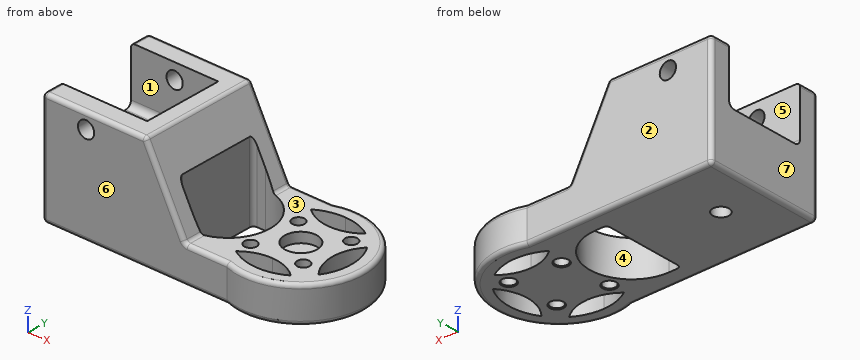
from build123d import *

# Parameters (mm, degrees)
ESQUISSE4_R                   = 13.9
ESQUISSE4_R_2                 = 1.55
BOSS_EXTRU_3_DEPTH            = 4.5
ESQUISSE7_R                   = 15.9
ESQUISSE7_R_2                 = 13.9
BOSS_EXTRU_7_DEPTH            = 9
BOSS_EXTRU_8_DEPTH            = 30
ENL_V_START                   = -4.5
ENL_V_MAT_EXTRU_12_OUTLINE_R  = 1.55
ENL_V_MAT_EXTRU_12_DEPTH      = 9
TROU_TARAUD_M32_D             = 2.5
TROU_TARAUD_M32_DEPTH         = 36
TROU_TARAUD_M32_CSINK_D       = 3.5
TROU_TARAUD_M32_CSINK_ANGLE   = 90
ENL_V_MAT_EXTRU_1_DEPTH       = 22
ESQUISSE13_R                  = 2.05
ENL_V_MAT_EXTRU_4_DEPTH       = 69.045108798
ESQUISSE15_R                  = 2.05
ENL_V_MAT_EXTRU_5_DEPTH       = 66.052954056
ENL_V_MAT_EXTRU_6_DEPTH       = 77.342234353
ESQUISSE24_R                  = 4.05
ENL_V_MAT_EXTRU_9_DEPTH       = 2.5
TROU_TARAUD_M33_D             = 2.5
TROU_TARAUD_M33_DEPTH         = 28.24245014
TROU_TARAUD_M33_CSINK_D       = 3.5
TROU_TARAUD_M33_CSINK_ANGLE   = 90
CONG_2_R                      = 1
ENL_V_MAT_EXTRU_13_DEPTH      = 58.499206362
ENL_V_MAT_EXTRU_13_DEPTH_BACK = 58.499206362
CONG_3_R                      = 1
CONG_4_R                      = 1


# Read off the part's stored shape, not the designer's step: Enlèv. mat.-Extru.12
with BuildPart() as part:
    # Esquisse4 → Boss.-Extru.3 (new, symmetric)
    with BuildSketch(Plane.XY):
        Circle(ESQUISSE4_R)
        with Locations((-6.717514421, -6.717514421)):
            Circle(ESQUISSE4_R_2, mode=Mode.SUBTRACT)
        with Locations((6.717514421, 6.717514421)):
            Circle(ESQUISSE4_R_2, mode=Mode.SUBTRACT)
        with Locations((-5.656854249, 5.656854249)):
            Circle(ESQUISSE4_R_2, mode=Mode.SUBTRACT)
        with Locations((5.656854249, -5.656854249)):
            Circle(ESQUISSE4_R_2, mode=Mode.SUBTRACT)
        with BuildLine():
            ThreePointArc((-10.594734512, 6.911881121), (-12.65, 0), (-10.594734512, -6.911881121))
            ThreePointArc((-10.594734512, -6.911881121), (-7.999175124, 0), (-10.594734512, 6.911881121))
        make_face(mode=Mode.SUBTRACT)
        with BuildLine():
            ThreePointArc((6.911881121, -10.594734512), (0, -7.999175124), (-6.911881121, -10.594734512))
            ThreePointArc((-6.911881121, -10.594734512), (0, -12.65), (6.911881121, -10.594734512))
        make_face(mode=Mode.SUBTRACT)
        with BuildLine():
            ThreePointArc((-6.911881121, 10.594734512), (0, 7.999175124), (6.911881121, 10.594734512))
            ThreePointArc((6.911881121, 10.594734512), (0, 12.65), (-6.911881121, 10.594734512))
        make_face(mode=Mode.SUBTRACT)
        with BuildLine():
            ThreePointArc((10.594734512, 6.911881121), (7.999175124, 0), (10.594734512, -6.911881121))
            ThreePointArc((10.594734512, -6.911881121), (12.65, 0), (10.594734512, 6.911881121))
        make_face(mode=Mode.SUBTRACT)
    extrude(amount=BOSS_EXTRU_3_DEPTH, both=True)

    # Esquisse7 → Boss.-Extru.7 (add)
    with BuildSketch(Plane.XY.offset(4.5)):
        Circle(ESQUISSE7_R)
        Circle(ESQUISSE7_R_2, mode=Mode.SUBTRACT)
    extrude(amount=-BOSS_EXTRU_7_DEPTH)

    # Esquisse6 → Boss.-Extru.8 (add)
    with BuildSketch(Plane(origin=(0, -15, 0), x_dir=(1, 0, 0), z_dir=(0, 1, 0))):
        Polygon((-51.798424989, -31.5), (-29.798424989, -31.5), (-15.9, -4.5), (0, -4.5), (0, 4.5), (-15.9, 4.5), (-51.798424989, 4.5), align=None)
    extrude(amount=BOSS_EXTRU_8_DEPTH)

    # Enlèv. mat.-Extru.12 outline → Enlèv. mat.-Extru.12 (cut)
    with BuildSketch(Plane.XY.offset(ENL_V_START)):
        with BuildLine():
            ThreePointArc((0, 12.65), (-3.605489456, 12.125301884), (-6.911881121, 10.594734512))
            ThreePointArc((-6.911881121, 10.594734512), (-6.773099648, 10.475509721), (-6.632262004, 10.358720998))
            ThreePointArc((-6.632262004, 10.358720998), (-6.631896353, 10.3589551), (-6.631530694, 10.359189189))
            ThreePointArc((-6.631530694, 10.359189189), (-3.519338467, 8.607363508), (0, 8))
            Line((0, 8), (0, 12.65))
        make_face()
        with BuildLine():
            ThreePointArc((-6.911881121, -10.594734512), (-3.605489456, -12.125301884), (0, -12.65))
            Line((0, -12.65), (0, -8))
            ThreePointArc((0, -8), (-3.519338467, -8.607363508), (-6.631530694, -10.359189189))
            ThreePointArc((-6.631530694, -10.359189189), (-6.631896353, -10.3589551), (-6.632262004, -10.358720998))
            ThreePointArc((-6.632262004, -10.358720998), (-6.773099648, -10.475509721), (-6.911881121, -10.594734512))
        make_face()
        with BuildLine():
            ThreePointArc((-10.358720998, 6.632262004), (-10.475509721, 6.773099648), (-10.594734512, 6.911881121))
            ThreePointArc((-10.594734512, 6.911881121), (-12.65, 0), (-10.594734512, -6.911881121))
            ThreePointArc((-10.594734512, -6.911881121), (-10.475509721, -6.773099648), (-10.358720998, -6.632262004))
            ThreePointArc((-10.358720998, -6.632262004), (-10.3589551, -6.631896353), (-10.359189189, -6.631530694))
            ThreePointArc((-10.359189189, -6.631530694), (-8, 0), (-10.359189189, 6.631530694))
            ThreePointArc((-10.359189189, 6.631530694), (-10.3589551, 6.631896353), (-10.358720998, 6.632262004))
        make_face()
        with Locations((-6.717514421, -6.717514421)):
            Circle(ENL_V_MAT_EXTRU_12_OUTLINE_R)
        with Locations((-5.656854249, 5.656854249)):
            Circle(ENL_V_MAT_EXTRU_12_OUTLINE_R)
    extrude(amount=ENL_V_MAT_EXTRU_12_DEPTH, mode=Mode.SUBTRACT)

    # Trou taraudé M32
    with Locations(Plane(origin=(5.656854249, -5.656854249, -4.5), x_dir=(-1, 0, 0), z_dir=(0, 0, -1))):
        with Locations((0, 0), (-1.060660172, 12.37436867)):
            CounterSinkHole(TROU_TARAUD_M32_D / 2, TROU_TARAUD_M32_CSINK_D / 2, depth=TROU_TARAUD_M32_DEPTH, counter_sink_angle=TROU_TARAUD_M32_CSINK_ANGLE)

    # Esquisse8 → Enlèv. mat.-Extru.1 (cut)
    with BuildSketch(Plane.ZY.offset(51.798424989)):
        with BuildLine():
            Line((28.34, 10.05), (11.34, 10.05))
            ThreePointArc((11.34, 10.05), (10.279339828, 9.610660172), (9.84, 8.55))
            Line((9.84, 8.55), (9.84, -8.55))
            ThreePointArc((9.84, -8.55), (10.279339828, -9.610660172), (11.34, -10.05))
            Line((11.34, -10.05), (28.34, -10.05))
            ThreePointArc((28.34, -10.05), (29.400660172, -9.610660172), (29.84, -8.55))
            Line((29.84, -8.55), (29.84, 8.55))
            ThreePointArc((29.84, 8.55), (29.400660172, 9.610660172), (28.34, 10.05))
        make_face()
    extrude(amount=-ENL_V_MAT_EXTRU_1_DEPTH, mode=Mode.SUBTRACT)

    # Esquisse13 → Enlèv. mat.-Extru.4 (cut, through all)
    with BuildSketch(Plane.XZ.offset(15)):
        with Locations(Location((-40.798424989, 19.84, 0), (0, 0, 270))):
            Circle(ESQUISSE13_R)
    extrude(amount=-ENL_V_MAT_EXTRU_4_DEPTH, mode=Mode.SUBTRACT)

    # Esquisse15 → Enlèv. mat.-Extru.5 (cut, through all)
    with BuildSketch(Plane(origin=(0, 0, -4.5), x_dir=(-1, 0, 0), z_dir=(0, 0, -1))):
        with Locations((40.798424989, 0)):
            Circle(ESQUISSE15_R)
    extrude(amount=-ENL_V_MAT_EXTRU_5_DEPTH, mode=Mode.SUBTRACT)

    # Esquisse16 → Enlèv. mat.-Extru.6 (cut, through all)
    with BuildSketch(Plane.ZY.offset(51.798424989)):
        Polygon((23.74245014, 10.05), (23.74245014, -10.05), (23.74245014, -15), (31.5, -15), (31.5, 15), (23.74245014, 15), align=None)
    extrude(amount=-ENL_V_MAT_EXTRU_6_DEPTH, mode=Mode.SUBTRACT)

    # Esquisse24 → Enlèv. mat.-Extru.9 (cut)
    with BuildSketch(Plane.XY.offset(4.5)):
        Circle(ESQUISSE24_R)
    extrude(amount=-ENL_V_MAT_EXTRU_9_DEPTH, mode=Mode.SUBTRACT)

    # Trou taraudé M33
    with Locations(Plane(origin=(0, 0, -4.5), x_dir=(-1, 0, 0), z_dir=(0, 0, -1))):
        with Locations((6.717514421, -6.717514421), (5.656854249, 5.656854249)):
            CounterSinkHole(TROU_TARAUD_M33_D / 2, TROU_TARAUD_M33_CSINK_D / 2, depth=TROU_TARAUD_M33_DEPTH, counter_sink_angle=TROU_TARAUD_M33_CSINK_ANGLE)

    # Congé2
    cong_2_edges = [part.edges().sort_by_distance(p)[0] for p in [
        (-20.852587961, -15, 14.12122507),
        (-20.852587961, 15, 14.12122507),
        (-38.801800455, 15, 23.74245014),
        (-25.805175921, 0, 23.74245014),
        (-38.801800455, -15, 23.74245014),
        (15.9, 0, -4.5),
        (15.9, 0, 4.5),
        (-15.9, 0, 4.5),
        (-10.586759375, -15, 4.5),
        (-28.535971869, -15, -4.5),
        (-51.798424989, 0, -4.5),
        (-28.535971869, 15, -4.5),
        (-10.586759375, 15, 4.5),
    ]]
    fillet(cong_2_edges, radius=CONG_2_R)

    # Esquisse27 → Enlèv. mat.-Extru.13 (cut, two sides: drawn at the far end of the back side and taken through both)
    with BuildSketch(Plane.XY.offset(4.5).offset(-ENL_V_MAT_EXTRU_13_DEPTH_BACK)):
        with BuildLine():
            Line((-18.31885198, -10.5), (-21.396528806, -10.5))
            Line((-21.396528806, -10.5), (-21.396528806, 10.5))
            Line((-21.396528806, 10.5), (-18.31885198, 10.5))
            ThreePointArc((-18.31885198, 10.5), (-7.81885198, 0), (-18.31885198, -10.5))
        make_face()
    extrude(amount=ENL_V_MAT_EXTRU_13_DEPTH + ENL_V_MAT_EXTRU_13_DEPTH_BACK, mode=Mode.SUBTRACT)

    # Congé3
    cong_3_edges = [part.edges().sort_by_distance(p)[0] for p in [
        (-21.396528806, 10.5, 5.338960274),
        (-21.396528806, -10.5, 5.338960274),
    ]]
    fillet(cong_3_edges, radius=CONG_3_R)

    # Congé4
    # the kernel refuses this fillet: 1 mm, written as the material it takes off along each edge
    with BuildSketch(Plane(origin=(-50.798424989, 14, -3.5), x_dir=(-1, 0, 0), z_dir=(0, 1, 0))) as cong_4_piece_1_section:
        Polygon((0, 0), (CONG_4_R, 0), (CONG_4_R, -CONG_4_R), (0, -CONG_4_R), align=None)
    cong_4_piece_1 = extrude(amount=CONG_4_R, mode=Mode.PRIVATE)
    cong_4_piece_1 = cong_4_piece_1 - Plane(origin=(-50.798424989, 14, -3.5), x_dir=(0.7071067811865477, 0, 0.7071067811865475), z_dir=(0, 1, 0)) * Sphere(CONG_4_R, mode=Mode.PRIVATE)
    add(cong_4_piece_1, mode=Mode.SUBTRACT)
    with BuildSketch(Plane(origin=(-50.798424989, -14, -3.5), x_dir=(-1, 0, 0), z_dir=(0, -1, 0))) as cong_4_piece_2_section:
        Polygon((0, 0), (CONG_4_R, 0), (CONG_4_R, CONG_4_R), (0, CONG_4_R), align=None)
    cong_4_piece_2 = extrude(amount=CONG_4_R, mode=Mode.PRIVATE)
    cong_4_piece_2 = cong_4_piece_2 - Plane(origin=(-50.798424989, -14, -3.5), x_dir=(0.7071067811865477, 0, 0.7071067811865475), z_dir=(0, -1, 0)) * Sphere(CONG_4_R, mode=Mode.PRIVATE)
    add(cong_4_piece_2, mode=Mode.SUBTRACT)
    with BuildSketch(Plane(origin=(-51.798424989, -14, 23.74245014), x_dir=(1, 0, 0), z_dir=(0, 1, 0)), Plane(origin=(-51.798424989, 7.55, 23.74245014), x_dir=(1, 0, 0), z_dir=(0, 1, 0))) as cong_4_piece_3:
        with BuildLine():
            CenterArc((CONG_4_R, CONG_4_R), CONG_4_R, 180, 90)
            Line((0, CONG_4_R), (0, 0))
            Line((0, 0), (CONG_4_R, 0))
        make_face()
    extrude(amount=6.45, mode=Mode.SUBTRACT)
    with BuildSketch(Plane(origin=(-51.798424989, -15, -3.5), x_dir=(1, 0, 0), z_dir=(0, 0, 1))) as cong_4_piece_4:
        with BuildLine():
            CenterArc((CONG_4_R, CONG_4_R), CONG_4_R, 180, 90)
            Line((0, CONG_4_R), (0, 0))
            Line((0, 0), (CONG_4_R, 0))
        make_face()
    extrude(amount=26.24245014, mode=Mode.SUBTRACT)
    with BuildSketch(Plane(origin=(-51.798424989, 15, -3.5), x_dir=(1, 0, 0), z_dir=(0, 0, 1))) as cong_4_piece_5:
        with BuildLine():
            CenterArc((CONG_4_R, -CONG_4_R), CONG_4_R, 90, 90)
            Line((0, -CONG_4_R), (0, 0))
            Line((0, 0), (CONG_4_R, 0))
        make_face()
    extrude(amount=26.24245014, mode=Mode.SUBTRACT)
    with BuildSketch(Plane(origin=(-51.798424989, 14, 22.74245014), x_dir=(0, 0, 1), z_dir=(0, -1, 0))) as cong_4_piece_6:
        with BuildLine():
            CenterArc((1 - CONG_4_R, -CONG_4_R), CONG_4_R, 0, 90)
            Line((1, -CONG_4_R), (1, 0))
            Line((1, 0), (1 - CONG_4_R, 0))
        make_face()
    revolve(axis=Axis((-51.798424989, 14, 22.74245014), (-1, 0, 0)), revolution_arc=90, mode=Mode.SUBTRACT)
    with BuildSketch(Plane(origin=(-51.798424989, -14, 22.74245014), x_dir=(0, 0, 1), z_dir=(0, 1, 0))) as cong_4_piece_7:
        with BuildLine():
            CenterArc((1 - CONG_4_R, CONG_4_R), CONG_4_R, 270, 90)
            Line((1 - CONG_4_R, 0), (1, 0))
            Line((1, 0), (1, CONG_4_R))
        make_face()
    revolve(axis=Axis((-51.798424989, -14, 22.74245014), (1, 0, 0)), revolution_arc=90, mode=Mode.SUBTRACT)


solid = part.part
Can you work these out from the model? Positions are in its coordinate system, mm. Face numbers are marked on the shaded views. A direction names the side the tool comes from. Give positions to 0.01 mm unless a question says otherwise; leave off trailing zeros. Loops run counter-clockwise (first coordinate to the right, second up) from the corner with the lowest first, then second, coordinate; pieces in that order, holes last. Notation, with made-up numbers: (22, -12.5) -> (45, -12.5) arc R25 cw to (45, 9.5) -> close; hole circle Ø1 at (-6.5, 10). An arc over 180 degrees is marked (long way). Write item = value, one per line.
1) I need wall thicknesses on L1, parallel to X at y = 4.5, z = -1.25; L2, parallel to Y at x = 6, z = 1.5; L3, parallel to Y at x = -39.5, z = 12. Which ranges of each line are inside material? Lowest first, please. Write a range as from..to.
Check result:
L1 = -51.8..-21.4, -8.83..-6.69, -4.63..9.01, 11.82..15.25
L2 = -14.72..-11.14, -9.88..-7.17, -4.15..5.34, 8.09..9.88, 11.14..14.72
L3 = -15..-10.05, 10.05..15
2) Suppose I cut it at B-B on x = -13. Write out the boundary of the cut face in (y, z).
Check result:
outline = (-15, -3.5) arc R1 ccw to (-14, -4.5) -> (-9.05, -4.5) -> (-9.05, 4.5) -> (-14, 4.5) arc R1 ccw to (-15, 3.5) -> close; (9.05, -4.5) -> (14, -4.5) arc R1 ccw to (15, -3.5) -> (15, 3.5) arc R1 ccw to (14, 4.5) -> (9.05, 4.5) -> close
3) Will these pins go through, and if not, where does the flat tip stop? pin 1 (7 mm diameter, centred on y = 4.5, z = 13.5, fed in from -X); pin 2 (15 mm diameter, centred on y = 1, z = 3.5, fed in from +X); pin 3 (13.5 mm diameter, centred on x = -36, z = 19, fed in from +Y); pin 4 (2.5 mm diameter, centred on x = 1, y = 1.5, fed in from +Z).
Check result:
pin_1 = -29.8
pin_2 = 15.9
pin_3 = 15
pin_4 = 2
4) For the marked faces 1, 2, 3 and 4, which set-ups out of +Z, -Z, +X, -X, +Y, -Y let a thin tool reach every point of the face, with its end or its side?
Check result:
face_1 = +Z, -X
face_2 = +Z, -Z, -X, +Y
face_3 = +Z, +X, +Y, -Y
face_4 = +Z, -Z
5) Thinking about a two-plate mould opening in Y: for the marked faces 5, 6 and 7, which applies, released by +Y, released by -Y, zero draft, split by the parting line, or undercut?
Check result:
face_5 = undercut
face_6 = released by -Y
face_7 = zero draft
6) Suppose I cut it at A-A on y = 0. Write out the boundary of the cut face in (x, z), then the cut area to 3 significant figures.
Check result:
outline = (-51.8, -3.5) arc R1 ccw to (-50.8, -4.5) -> (-42.85, -4.5) -> (-42.85, 9.84) -> (-51.8, 9.84) -> close; (-38.75, -4.5) -> (-21.4, -4.5) -> (-21.4, 15.18) -> (-25.53, 23.2) arc R1 ccw to (-26.42, 23.74) -> (-29.8, 23.74) -> (-29.8, 9.84) -> (-38.75, 9.84) -> close; (-7.82, -4.5) -> (8, -4.5) -> (8, 4.5) -> (4.05, 4.5) -> (4.05, 2) -> (-4.05, 2) -> (-4.05, 4.5) -> (-7.82, 4.5) -> close; (12.65, -4.5) -> (14.9, -4.5) arc R1 ccw to (15.9, -3.5) -> (15.9, 3.5) arc R1 ccw to (14.9, 4.5) -> (12.65, 4.5) -> close
area = 626 mm2
7) Suppose I cut it at C-C on z = 19.84. Give the number of separate pieces and of enclosed holes in the cut face, then the cut area to 3 significant figures.
Check result:
separate_pieces = 3
enclosed_holes = 0
area = 356 mm2
